Work out the finished part from the listing and answer in its coordinate system (mm). A direction names the side the tool comes from. Give positions to 0.01 mm unless a question says otherwise; leave off trailing zeros. Loops run counter-clockwise (first coordinate to the right, second up) from the corner with the lowest first, then second, coordinate; pieces in that order, holes last. Notation, with made-up numbers: M -5,58 L 4,58 A17 ccw 4,90 Z; hole C -11,29.5 d1. An arc over 180 degrees is marked long. Use a Markdown table: item, result.
Autodesk Inventor part; units mm, degrees
ref_plane "YZ Plane" through (0, 0, 0) normal (1, 0, 0) x (0, 1, 0)
ref_plane "XZ Plane" through (0, 0, 0) normal (0, 1, 0) x (-1, 0, 0)
ref_plane "XY Plane" through (0, 0, 0) normal (0, 0, 1) x (1, 0, 0)
sketch "Sketch2" plane through (0, 0, 0) normal (0, 1, 0) x (-1, 0, 0)
  line L0 (0, 0) -> (-20, 0)
  line L1 (-20, 0) -> (-20, -20)
  line L2 (-20, -20) -> (0, -20)
  line L3 (0, -20) -> (0, 0)
  dimension "d0" = 20
  dimension "d1" = 20
extrude "Extrusion1" add sketch "Sketch2" along normal blind 1.5
sketch "Sketch3" plane through (0, 1.5, 0) normal (0, 1, 0) x (1, 0, 0)
  circle A0 centre (3.8617, 4.2192) radius 3
  circle A1 centre (13.0724, 4.7341) radius 3.05
  circle A2 centre (3.8617, 14.7744) radius 3.075
  circle A3 centre (13.0724, 14.946) radius 3.125
  point P0 (0, 0)
  dimension "d4" = 6
  dimension "d5" = 6.1
  dimension "d6" = 6.15
  dimension "d7" = 6.25
extrude "Extrusion2" add sketch "Sketch3" along normal blind 3
fillet "Fillet1" radius 1 4 edges at (10.0224, 1.5, -4.7341) (0.8617, 1.5, -4.2192) (0.7867, 1.5, -14.7744) (9.9474, 1.5, -14.946)
chamfer "Chamfer1" distance 0.5 angle 45 4 edges at (10.0224, 4.5, -4.7341) (9.9474, 4.5, -14.946) (0.7867, 4.5, -14.7744) (0.8617, 4.5, -4.2192)
properties part number "heligearPressFitTester"
(1) A cutting plane is placed at B-B (x = 8.25). Write down the section's boundary in (y, z).
Entries:
| item | result |
|---|---|
| outline | M 0,-20 L 1.5,-20 L 1.5,0 L 0,0 Z |
(2) The mould has two halves that part along X. Classify faces 3 (the flat face through (10, 1, 0)), 4 (the cylindrical face through (3.195, 3.228, -17.776)), 5 (the cylindrical face through (10.025, 3.24, -4.6)), 6 (the flat face through (0, 1, -10)): released by +X, released by -X, zero draft, split by the parting line, or undercut.
Entries:
| item | result |
|---|---|
| face 3 | zero draft |
| face 4 | undercut |
| face 5 | undercut |
| face 6 | released by -X |
(3) Which of the six approach directions +Z, -Z, +X, -X, +Y, -Y give full straight-line access (tool end or side, diameter ignored) to faces 1 (the cylindrical face through (6.723, 3.235, -3.318)), 2 (the flat face through (4, 4.5, -4))?
Entries:
| item | result |
|---|---|
| face 1 | +Y |
| face 2 | +Z, -Z, +X, -X, +Y |
(4) Given P1, Ø4, axis at x = 8.5, z = -7.5, coming from the +Y side, flat-ended and moving along its own axis, determine where the tip first touches the part or whether it passes through.
Entries:
| item | result |
|---|---|
| P1 | stops at y = 1.79 |
(5) A cutting plane is placed at A-A (y = 4.25). Write down the section's boundary in (x, z) (3 decimals).
Entries:
| item | result |
|---|---|
| outline | C 3.862,-14.774 d5.65; C 3.862,-4.219 d5.5; C 13.072,-14.946 d5.75; C 13.072,-4.734 d5.6 |
(6) A cutting plane is placed at C-C (y = 1.9). Count the separate pieces of the cut face and the enclosed holes in it, and give its area (3 significant figures).
Entries:
| item | result |
|---|---|
| separate pieces | 4 |
| enclosed holes | 0 |
| area | 134 mm² |
(7) Consider probe 1 along Y at (x, z) = (7.5, -17.25); probe 2 along Z at (x, y) = (12.5, 3.7); probe 3 along Z at (x, y) = (12.75, 3). Determine where each line is inside the solid, lowest interval first. Write a range as [from, to].
Entries:
| item | result |
|---|---|
| probe 1 | y = [0, 1.5] |
| probe 2 | z = [-18.02, -11.87], [-7.73, -1.74] |
| probe 3 | z = [-18.05, -11.84], [-7.77, -1.7] |
